from build123d import *

# Parameters (mm, degrees)
SKETCH_1_R      = 0.35
EXTRUDE_1_DEPTH = 8


with BuildPart() as part:
    # 草图1 → 凸台-拉伸1 (new body)
    with BuildSketch(Plane(origin=(0, 0, 0), x_dir=(0, 0, -1), z_dir=(1, 0, 0))):
        with BuildLine():
            Line((0.3, -1.058300524), (0.3, -9.058300524))
            Line((0.3, -9.058300524), (-0.3, -9.058300524))
            Line((-0.3, -9.058300524), (-0.3, -1.058300524))
            ThreePointArc((-0.3, -1.058300524), (0, 1.1), (0.3, -1.058300524))
        make_face()
        Circle(SKETCH_1_R, mode=Mode.SUBTRACT)
    extrude(amount=EXTRUDE_1_DEPTH)


solid = part.part
Input: part model. Units: mm. Frame: model coordinates. A direction names the side the tool comes from. Coordinates: 2 decimals unless noted, no trailing zeros. Loops run counter-clockwise (first coordinate to the right, second up) from the corner with the lowest first, then second, coordinate; pieces in that order, holes last.
(1) Section C-C on x = 6. Return the cut outline in (y, z).
(2) First-contact query: pin 1 Ø1.5 at (x, y) = (6, -2.5) entering from -Z. Flat tip, straight axial feed; report the tip coordinate or a pass-through.
(3) Set-up query: faces 1 (the face through (4, -5, 0.3)), 2 (the face through (4, -5, -0.3)), 3 (the face through (0, -3, 0)). Return all of +Z, -Z, +X, -X, +Y, -Y with unobstructed straight access to the full face (end or side cutting, diameter ignored); none if empty.
(4) Section B-B on y = 0. Return the cut outline in (x, z), then the cut area to 3 significant figures.
(5) Section A-A on z = 0. Return the cut outline in (x, y), then the cut area to 3 significant figures.
(6) Section D-D on y = -4.25. Return the cut outline in (x, z).
(7) Material intervals for probe 1 along Y at (x, z) = (2.25, -0.05); probe 2 along Z at (x, y) = (5.75, -4.75); probe 3 along Z at (x, y) = (6.5, -0.25), sorted ascending.
Data:
1. outline: (-9.06, -0.3) - (-1.06, -0.3) arc R1.1 ccw (long way) to (-1.06, 0.3) - (-9.06, 0.3) - close; hole circle Ø0.7 at (0, 0)
2. pin 1: stops at z = -0.3
3. face 1: +Z, +X, -X, -Y
3. face 2: -Z, +X, -X, -Y
3. face 3: +Z, -Z, -X, +Y, -Y
4. outline: (0, -1.1) - (8, -1.1) - (8, -0.35) - (0, -0.35) - close; (0, 0.35) - (8, 0.35) - (8, 1.1) - (0, 1.1) - close
4. area: 12.0 mm2
5. outline: (0, -9.06) - (8, -9.06) - (8, -0.35) - (0, -0.35) - close; (0, 0.35) - (8, 0.35) - (8, 1.1) - (0, 1.1) - close
5. area: 75.7 mm2
6. outline: (0, -0.3) - (8, -0.3) - (8, 0.3) - (0, 0.3) - close
7. probe 1: y = -9.06 to -0.35, 0.35 to 1.1
7. probe 2: z = -0.3 to 0.3
7. probe 3: z = -1.07 to -0.24, 0.24 to 1.07
